from build123d import *

# Parameters (mm, degrees)
SKETCH1_W             = 20.828
SKETCH1_H             = 20.828
BOSS_EXTRUDE1_DEPTH   = 38.1
SKETCH1_W_2           = 39.116
SKETCH1_H_2           = 39.116
SKETCH1_W_3           = 26.416
SKETCH1_H_3           = 26.416
BOSS_EXTRUDE1_2_DEPTH = 38.1
SKETCH2_R             = 1.9558
CUT_EXTRUDE1_DEPTH    = 59.001610495
SKETCH1_2_W           = 39.116
SKETCH1_2_H           = 39.116
SKETCH1_2_W_2         = 26.416
SKETCH1_2_H_2         = 26.416
SKETCH1_2_W_3         = 20.828
SKETCH1_2_H_3         = 20.828
BOSS_EXTRUDE2_DEPTH   = 6.35
FILLET1_R             = 2.54


with BuildPart() as part:
    # Sketch1 → Boss-Extrude1 (new body)
    with BuildSketch(Plane(origin=(0, 0, 0), x_dir=(1, 0, 0), z_dir=(0, 1, 0))):
        Rectangle(SKETCH1_W, SKETCH1_H)
    extrude(amount=BOSS_EXTRUDE1_DEPTH)


with BuildPart() as body_2:
    # Sketch1 → Boss-Extrude1 2 (new body)
    with BuildSketch(Plane(origin=(0, 0, 0), x_dir=(1, 0, 0), z_dir=(0, 1, 0))):
        Rectangle(SKETCH1_W_2, SKETCH1_H_2)
        Rectangle(SKETCH1_W_3, SKETCH1_H_3, mode=Mode.SUBTRACT)
    extrude(amount=BOSS_EXTRUDE1_2_DEPTH)


with BuildPart() as cut_extrude1_tool:
    # Sketch2 → Cut-Extrude1 (new, through all)
    with BuildSketch(Plane.XY.offset(19.558)):
        with Locations((-7.239, 30.226)):
            Circle(SKETCH2_R)
        with Locations((7.239, 30.226)):
            Circle(SKETCH2_R)
        with Locations((7.239, 4.826)):
            Circle(SKETCH2_R)
        with Locations((-7.239, 4.826)):
            Circle(SKETCH2_R)
    extrude(amount=-CUT_EXTRUDE1_DEPTH)


with BuildPart() as part_1:
    add(part.part)

    # Cut-Extrude1: cut by cut_extrude1_tool
    add(cut_extrude1_tool.part, mode=Mode.SUBTRACT)



with BuildPart() as body_2_1:
    add(body_2.part)

    # Cut-Extrude1: cut by cut_extrude1_tool
    add(cut_extrude1_tool.part, mode=Mode.SUBTRACT)


with BuildPart() as part_2:
    add(part_1.part)

    add(body_2_1.part)  # Boss-Extrude2 merges body 2
    # Sketch1<2> → Boss-Extrude2 (add)
    # profile 1 of 3: a face of its own
    with BuildSketch(Plane(origin=(0, 0, 0), x_dir=(1, 0, 0), z_dir=(0, 1, 0))):
        Rectangle(SKETCH1_2_W, SKETCH1_2_H)
        Rectangle(SKETCH1_2_W_2, SKETCH1_2_H_2, mode=Mode.SUBTRACT)
    # profile 2 of 3: a face of its own
    with BuildSketch(Plane(origin=(0, 0, 0), x_dir=(1, 0, 0), z_dir=(0, 1, 0))):
        Rectangle(SKETCH1_2_W_2, SKETCH1_2_H_2)
        Rectangle(SKETCH1_2_W_3, SKETCH1_2_H_3, mode=Mode.SUBTRACT)
    # profile 3 of 3: a face of its own
    with BuildSketch(Plane(origin=(0, 0, 0), x_dir=(1, 0, 0), z_dir=(0, 1, 0))):
        Rectangle(SKETCH1_2_W_3, SKETCH1_2_H_3)
    extrude(amount=-BOSS_EXTRUDE2_DEPTH)

    # Fillet1
    # the kernel refuses this fillet: 2.54 mm, written as the material it takes off along each edge
    with BuildSketch(Plane(origin=(-19.558, 44.45, -19.558), x_dir=(0, 0, 1), z_dir=(0, -1, 0)), Plane(origin=(-19.558, -12.7, 19.558), x_dir=(0, 0, -1), z_dir=(0, 1, 0))) as fillet1_piece_1:
        with BuildLine():
            CenterArc((FILLET1_R, -FILLET1_R), FILLET1_R, 90, 90)
            Line((0, -FILLET1_R), (0, 0))
            Line((0, 0), (FILLET1_R, 0))
        make_face()
    extrude(amount=57.15, mode=Mode.SUBTRACT)
    with BuildSketch(Plane(origin=(19.558, 44.45, -19.558), x_dir=(0, 0, 1), z_dir=(0, -1, 0)), Plane(origin=(19.558, -12.7, 19.558), x_dir=(0, 0, -1), z_dir=(0, 1, 0))) as fillet1_piece_2:
        with BuildLine():
            CenterArc((FILLET1_R, FILLET1_R), FILLET1_R, 180, 90)
            Line((0, FILLET1_R), (0, 0))
            Line((0, 0), (FILLET1_R, 0))
        make_face()
    extrude(amount=57.15, mode=Mode.SUBTRACT)
    with BuildSketch(Plane(origin=(10.414, 0, -10.414), x_dir=(-1, 0, 0), z_dir=(0, 1, 0)), Plane(origin=(-10.414, 0, -10.414), x_dir=(0, 0, 1), z_dir=(0, 1, 0))) as fillet1_piece_3:
        with BuildLine():
            CenterArc((FILLET1_R, FILLET1_R), FILLET1_R, 180, 90)
            Line((0, FILLET1_R), (0, 0))
            Line((0, 0), (FILLET1_R, 0))
        make_face()
    extrude(amount=44.45, mode=Mode.SUBTRACT)
    with BuildSketch(Plane(origin=(-10.414, 0, 10.414), x_dir=(0, 0, -1), z_dir=(0, 1, 0)), Plane(origin=(10.414, 0, 10.414), x_dir=(-1, 0, 0), z_dir=(0, 1, 0))) as fillet1_piece_4:
        with BuildLine():
            CenterArc((FILLET1_R, -FILLET1_R), FILLET1_R, 90, 90)
            Line((0, -FILLET1_R), (0, 0))
            Line((0, 0), (FILLET1_R, 0))
        make_face()
    extrude(amount=44.45, mode=Mode.SUBTRACT)


solid = part_2.part
Here's how the part is built. I have some questions about the finished solid (model axes, mm). A direction names the side the tool comes from. Coordinates: 2 decimals unless noted, no trailing zeros. Write each loop counter-clockwise with the first axis right and the second up, starting at its lowest first coordinate (ties: lowest second). Pieces come first, ordered by that corner, then holes.
1) If we section it at C-C (z = 14): List the corners of the cut face in (x, y) for me.
Filled in:
outline: (-19.56, -6.35) - (19.56, -6.35) - (19.56, 38.1) - (-19.56, 38.1) - close; hole circle Ø3.91 at (-7.24, 4.83); hole circle Ø3.91 at (-7.24, 30.23); hole circle Ø3.91 at (7.24, 4.83); hole circle Ø3.91 at (7.24, 30.23)
2) If we section it at B-B (x = -1.5): List the corners of the cut face in (y, z) for me.
Filled in:
outline: (-6.35, -19.56) - (38.1, -19.56) - (38.1, -13.21) - (0, -13.21) - (0, -10.41) - (38.1, -10.41) - (38.1, 10.41) - (0, 10.41) - (0, 13.21) - (38.1, 13.21) - (38.1, 19.56) - (-6.35, 19.56) - close
3) Which directions (+Z, -Z, +X, -X, +Y, -Y) give clear straight access to the entire face, cutting with the end or side of a thin tool? Please do faces 1 (the face through (-6.188, 31.875, 16.427)), 2 (the face through (10.414, 19, 0)).
Filled in:
face 1: +Z, -Z
face 2: +Y
4) If we section it at D-D (z = -12.5): List the corners of the cut face in (x, y) for me, plus the area to 3 significant figures.
Filled in:
outline: (-19.56, -6.35) - (19.56, -6.35) - (19.56, 38.1) - (13.21, 38.1) - (13.21, 0) - (-13.21, 0) - (-13.21, 38.1) - (-19.56, 38.1) - close
area: 732 mm2
5) Thinking about a two-plate mould opening in Z: for faces 3 (the face through (0, 19, -10.414)), 4 (the face through (-5.374, 5.413, -16.339)), 5 (the face through (-9.69, 18.78, 9.65)), 6 (the face through (18.794, 16.186, -18.834)), which applies, +Z half, -Z half, draft (parallel to the pull), parting line (faces both ways), or undercut?
Filled in:
face 3: undercut
face 4: draft
face 5: undercut
face 6: -Z half
6) If I drill on line 1 (Z direction, x = 1, y = 20.5); line 2 (X direction, y = 30, z = -16), over which ranges is the centre line in solid material (lowest first)?
Filled in:
line 1: z = -19.56 to -13.21, -10.41 to 10.41, 13.21 to 19.56
line 2: x = -19.56 to -9.18, -5.3 to 5.3, 9.18 to 19.56
7) If we section it at A-A (y = 17.5): List the corners of the cut face in (x, z) for me.
Filled in:
outline: (-19.56, -17.02) arc R2.54 ccw to (-17.02, -19.56) - (17.02, -19.56) arc R2.54 ccw to (19.56, -17.02) - (19.56, 17.02) arc R2.54 ccw to (17.02, 19.56) - (-17.02, 19.56) arc R2.54 ccw to (-19.56, 17.02) - close; (-10.41, -7.87) arc R2.54 ccw to (-7.87, -10.41) - (7.87, -10.41) arc R2.54 ccw to (10.41, -7.87) - (10.41, 7.87) arc R2.54 ccw to (7.87, 10.41) - (-7.87, 10.41) arc R2.54 ccw to (-10.41, 7.87) - close; hole (-13.21, -13.21) - (13.21, -13.21) - (13.21, 13.21) - (-13.21, 13.21) - close
